Part model, mm, in its own coordinate system. Face numbers are marked on the shaded views. Give positions to 0.01 mm unless a question says otherwise; leave off trailing zeros. Order: outer loops, then holes, each group sorted by start corner. A loop starts at its lowest first (then second) coordinate and runs counter-clockwise, first axis right, second up. Notation, with made-up numbers: M 38.25,18.5 L 58.25,18.5 A24 cw 58.25,29.5 Z; hole C 36.25,56.25 d1. An arc over 180 degrees is marked long. Write each question's results on one line, items separated by ' | '. Start each with the question number.
Autodesk Inventor part; units mm, degrees
ref_plane "YZ Plane" through (0, 0, 0) normal (1, 0, 0) x (0, 1, 0)
ref_plane "XZ Plane" through (0, 0, 0) normal (0, 1, 0) x (-1, 0, 0)
ref_plane "XY Plane" through (0, 0, 0) normal (0, 0, 1) x (1, 0, 0)
sketch "Skizze1" plane through (0, 0, 0) normal (0, 1, 0) x (-1, 0, 0)
  line L0 (0, 11) -> (0, -11) construction
  line L1 (9.5, 0) -> (-9.5, 0) construction
  arc A0 (3.5777, 12.7889) -> (-3.5777, 12.7889) centre (0, 11) ccw
  arc A1 (-3.5777, -12.7889) -> (3.5777, -12.7889) centre (0, -11) ccw
  arc A2 (9.0777, -1.7889) -> (9.0777, 1.7889) centre (5.5, 0) ccw
  arc A3 (-9.0777, 1.7889) -> (-9.0777, -1.7889) centre (-5.5, 0) ccw
  line L2 (-3.5777, 12.7889) -> (-9.0777, 1.7889)
  line L3 (3.5777, -12.7889) -> (9.0777, -1.7889)
  line L4 (9.0777, 1.7889) -> (3.5777, 12.7889)
  line L5 (-9.0777, -1.7889) -> (-3.5777, -12.7889)
  point P0 (0, 0)
  point P1 (0, 0)
  point P2 (0, -15)
  point P3 (0, 15)
  dimension "d4" = 19
  dimension "d5" = 22
  dimension "d6" = 4
  dimension "d7" = 4
  dimension "d8" = 4
  dimension "d9" = 4
  dimension "d10" = 30
extrude "Extrusion1" add sketch "Skizze1" along normal blind 6
sketch "Skizze2" plane through (0, 6, 0) normal (0, 1, 0) x (1, 0, 0)
  arc A0 (-3.5777, -12.7889) -> (3.5777, -12.7889) centre (0, -11) ccw
  arc A1 (3.5777, 12.7889) -> (-3.5777, 12.7889) centre (0, 11) ccw
  point P0 (0, 0)
hole "Bohrung1" at (0, 6, 11) at (0, 6, -11) direction (0, -1, 0) diameter 4 depth 6
sketch "Skizze3" plane through (0, 6, 0) normal (0, 1, 0) x (1, 0, 0)
  point P0 (0, 0)
  point P1 (0, 0)
hole "Bohrung2" at (0, 6, 0) direction (0, -1, 0) diameter 10 end through all
equation "\"d6\" = d7"
equation "\"d9\" = d8"
properties part number "1162"
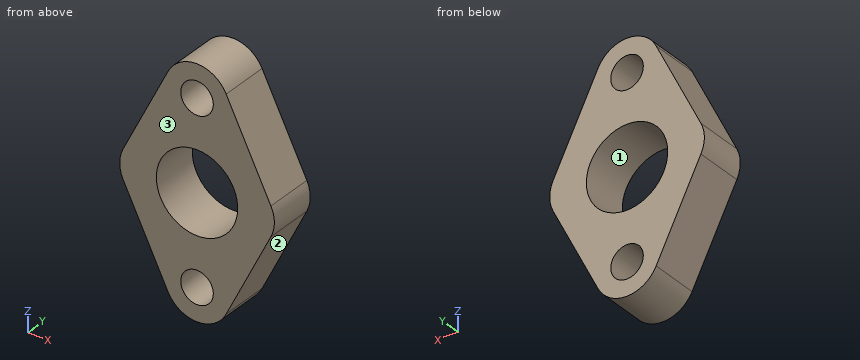
(1) Drop a flat-ended pin along its axis: P1, Ø3, axis at y = 5.5, z = 11.5, coming from the +X side. Give the stop position or say it passes through.
(2) Probe L1, parallel to X at y = 2.4, z = 0; L2, parallel to Z at x = 1, y = 3.55; L3, parallel to Z at x = -0.5, y = 5.25. List the from-to ranges inside material, lowest first.
(3) Saw through at C-C on y = 4.35. Give the cut face in (x, z).
(4) Saw through at B-B on x = 0. Give the cut face in (y, z), plus the area to 3 significant figures.
(5) Pull direction X, two halves, no side cores. Call the marked faces 1, 2 and 3: +X half, -X half, draft (parallel to the pull), parting line (faces both ways), or undercut.
(6) Saw through at D-D on z = 4. Give the cut face in (x, y), plus the area to 3 significant figures.
(7) Saw through at A-A on z = 0. Give the cut face in (x, y).
Taken from the geometry:
1) P1: stops at x = 4.97
2) L1: x = -9.5 to -5, 5 to 9.5 | L2: z = -14.87 to -12.73, -9.27 to -4.9, 4.9 to 9.27, 12.73 to 14.87 | L3: z = -14.97 to -12.94, -9.06 to -4.97, 4.97 to 9.06, 12.94 to 14.97
3) outline: M -9.08,-1.79 L -3.58,-12.79 A4 ccw 3.58,-12.79 L 9.08,-1.79 A4 ccw 9.08,1.79 L 3.58,12.79 A4 ccw -3.58,12.79 L -9.08,1.79 A4 ccw Z; hole C 0,0 d10; hole C 0,-11 d4; hole C 0,11 d4
4) outline: M 0,-15 L 6,-15 L 6,-13 L 0,-13 Z; M 0,-9 L 6,-9 L 6,-5 L 0,-5 Z; M 0,5 L 6,5 L 6,9 L 0,9 Z; M 0,13 L 6,13 L 6,15 L 0,15 Z | area: 72.0 mm²
5) face 1: undercut | face 2: +X half | face 3: draft
6) outline: M -7.97,0 L -3,0 L -3,6 L -7.97,6 Z; M 3,0 L 7.97,0 L 7.97,6 L 3,6 Z | area: 59.7 mm²
7) outline: M -9.5,0 L -5,0 L -5,6 L -9.5,6 Z; M 5,0 L 9.5,0 L 9.5,6 L 5,6 Z
